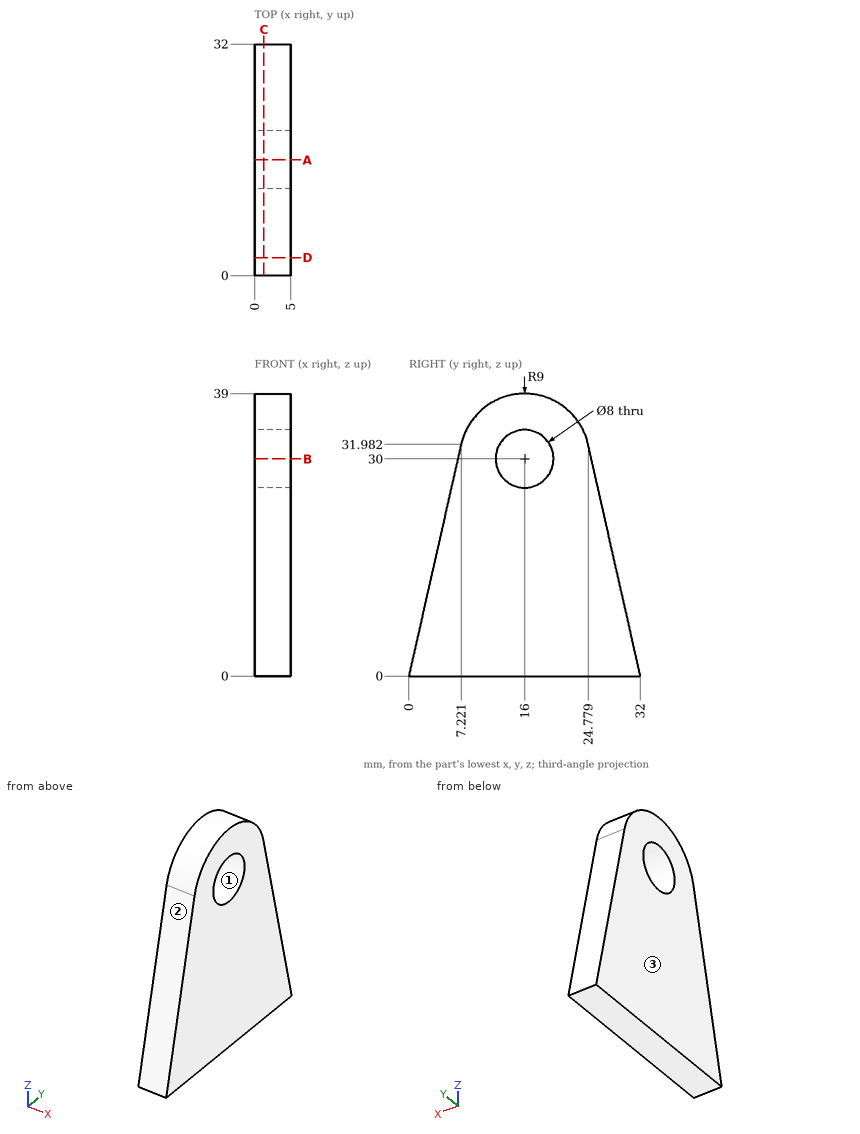
Answer from the drawing. Dimensions are ordinates in mm from the lowest x, y and z of the part. Round coordinates to 2 decimals unless told otherwise and drop trailing zeros. Order: outer loops, then holes, each group sorted by start corner. A loop starts at its lowest first (then second) coordinate and runs counter-clockwise, first axis right, second up.
1) The part is cut by section B-B on z = 30. Write down the section's boundary in (x, y), plus the area to 3 significant figures.
2) Straight lines are drawn through the part: L1, parallel to Z at x = 1.65, y = 17; L2, parallel to Y at x = 1.65, z = 30; L3, parallel to Y at x = 4.2, z = 31. For each, find the intervals that lie inside material, in ascending order.
3) The part is cut by section C-C on x = 1.3. Write down the section's boundary in (y, z), plus the area to 3 significant figures.
4) Flat-ended cylindrical pins translate along their axes: pin 1 (3 mm diameter, centred on x = 4.5, z = 5, fed in from -Y); pin 2 (1.5 mm diameter, centred on x = 2.5, z = 11, fed in from -Y). Find the tip coordinate at first contact, or state that the pin passes through.
5) The mould has two halves that part along Y. Classify the marked faces 1, 2 and 3: released by +Y, released by -Y, zero draft, split by the parting line, or undercut.
6) The part is cut by section D-D on y = 2.5. Write down the section's boundary in (x, z).
7) The part is cut by section A-A on y = 16. Write down the section's boundary in (x, z).
Resolved:
1. outline: (0, 6.77) - (5, 6.77) - (5, 12) - (0, 12) - close; (0, 20) - (5, 20) - (5, 25.23) - (0, 25.23) - close
1. area: 52.3 mm2
2. L1: z = 0 to 26.13, 33.87 to 38.94
2. L2: y = 6.77 to 12, 20 to 25.23
2. L3: y = 7 to 12.13, 19.87 to 25
3. outline: (0, 0) - (32, 0) - (24.78, 31.98) arc R9 ccw to (7.22, 31.98) - close; hole circle Ø8 at (16, 30)
3. area: 834 mm2
4. pin 1: stops at y = 0.79
4. pin 2: stops at y = 2.31
5. face 1: undercut
5. face 2: released by -Y
5. face 3: zero draft
6. outline: (0, 0) - (5, 0) - (5, 11.07) - (0, 11.07) - close
7. outline: (0, 0) - (5, 0) - (5, 26) - (0, 26) - close; (0, 34) - (5, 34) - (5, 39) - (0, 39) - close
